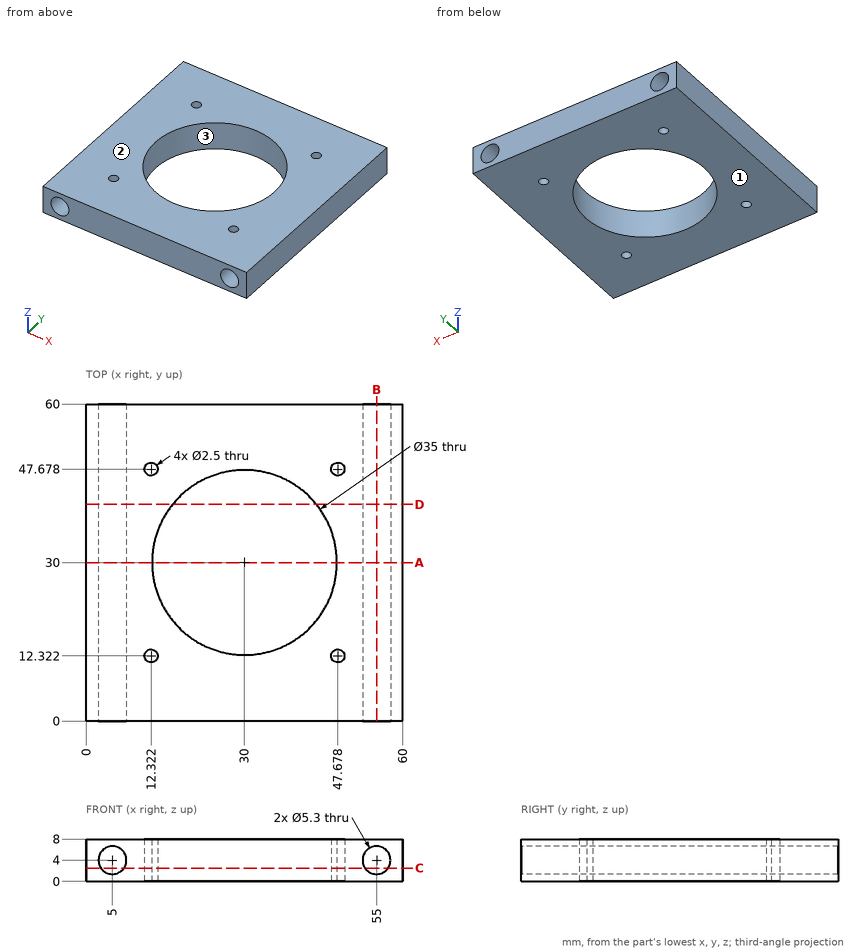
Here's the drawing with two shaded views (mm, measured from the low corner). I have some questions. Give positions to 0.01 mm unless a question says otherwise; leave off trailing zeros. Write each loop counter-clockwise with the first axis right and the second up, starting at its lowest first coordinate (ties: lowest second). Pieces come first, ordered by that corner, then holes. Notation, with made-up numbers: (49, 26.25) -> (95, 26.25) arc R28 ccw to (95, 52.25) -> close; hole circle Ø2 at (47, 57). An arc over 180 degrees is marked (long way). Use one line per item in the form item = value. Start each with the question number.
1. Imagine slicing it at D-D on y = 41. List the corners of the cut face in (x, z) for me.
2. Will this pin go through, and if not, where does the flat tip stop? pin 1 Ø3 at (x, y) = (12.32, 12.32) entering from +Z.
3. Imagine slicing it at B-B on x = 55. List the corners of the cut face in (y, z) for me, plus the area to 3 significant figures.
4. Imagine slicing it at C-C on z = 2.5. State how many separate pieces and enclosed holes the cut face has, plus the area to 3 significant figures.
5. Thinking about a two-plate mould opening in Z: for the marked faces 1, 2 and 3, which applies, +Z half, -Z half, draft (parallel to the pull), parting line (faces both ways), or undercut?
6. Imagine slicing it at A-A on y = 30. List the corners of the cut face in (x, z) for me, plus the area to 3 significant figures.
7. If I drill on L1, parallel to Y at x = 30, z = 5.75; L2, parallel to Y at x = 12, z = 1.5 (1 decimal); L3, parallel to X at y = 51.5, z = 5 (1 decimal), over which ranges is the centre line in solid material (lowest first)?
Entries:
q1.outline = (0, 0) -> (16.39, 0) -> (16.39, 8) -> (0, 8) -> close; (43.61, 0) -> (60, 0) -> (60, 8) -> (43.61, 8) -> close; hole circle Ø5.3 at (5, 4); hole circle Ø5.3 at (55, 4)
q2.pin_1 = 8
q3.outline = (0, 0) -> (60, 0) -> (60, 1.35) -> (0, 1.35) -> close; (0, 6.65) -> (60, 6.65) -> (60, 8) -> (0, 8) -> close
q3.area = 162 mm²
q4.separate_pieces = 3
q4.enclosed_holes = 5
q4.area = 2,090 mm²
q5.face_1 = -Z half
q5.face_2 = +Z half
q5.face_3 = draft
q6.outline = (0, 0) -> (12.5, 0) -> (12.5, 8) -> (0, 8) -> close; (47.5, 0) -> (60, 0) -> (60, 8) -> (47.5, 8) -> close; hole circle Ø5.3 at (5, 4); hole circle Ø5.3 at (55, 4)
q6.area = 156 mm²
q7.L1 = 0 to 12.5, 47.5 to 60
q7.L2 = 0 to 11.1, 13.5 to 46.5, 48.9 to 60
q7.L3 = 0 to 2.5, 7.5 to 52.5, 57.5 to 60
